Input: part model. Units: mm. Frame: model coordinates. Coordinates: 2 decimals unless noted, no trailing zeros. Loops run counter-clockwise (first coordinate to the right, second up) from the corner with the lowest first, then second, coordinate; pieces in that order, holes last. Notation, with made-up numbers: (68, -14.5) - (93, -14.5) arc R35 ccw to (93, 17.5) - close; hole circle Ø5 at (57.5, 44.5). An arc over 180 degrees is marked (long way). Use one line per item in the form item = value.
from build123d import *

# Parameters (mm, degrees)
BOSS_EXTRUDE1_DEPTH          = 1
CUT_EXTRUDE1_REACH           = 153.019
SKETCH2_R                    = 5.25
LPATTERN1_COUNT              = 6
LPATTERN1_PITCH              = 20
CIRPATTERN1_COPY_1_REACH     = 153.019
CIRPATTERN1_COPY_1_SKETCH_R  = 5.25
CIRPATTERN1_COPY_2_REACH     = 153.019
CIRPATTERN1_COPY_2_SKETCH_R  = 5.25
CIRPATTERN1_COPY_3_REACH     = 153.019
CIRPATTERN1_COPY_3_SKETCH_R  = 5.25
CIRPATTERN1_COPY_4_REACH     = 153.019
CIRPATTERN1_COPY_4_SKETCH_R  = 5.25
CIRPATTERN1_COPY_5_REACH     = 153.019
CIRPATTERN1_COPY_5_SKETCH_R  = 5.25
CIRPATTERN1_COPY_6_REACH     = 153.019
CIRPATTERN1_COPY_6_SKETCH_R  = 5.25
CIRPATTERN1_COPY_7_REACH     = 153.019
CIRPATTERN1_COPY_7_SKETCH_R  = 5.25
CIRPATTERN1_COPY_8_REACH     = 153.019
CIRPATTERN1_COPY_8_SKETCH_R  = 5.25
CIRPATTERN1_COPY_9_REACH     = 153.019
CIRPATTERN1_COPY_9_SKETCH_R  = 5.25
CIRPATTERN1_COPY_10_REACH    = 153.019
CIRPATTERN1_COPY_10_SKETCH_R = 5.25


with BuildPart() as part:
    # Sketch1 → Boss-Extrude1 (new, symmetric)
    with BuildSketch(Plane(origin=(0, 0, 0), x_dir=(1, 0, 0), z_dir=(0, 1, 0))):
        with BuildLine():
            ThreePointArc((-92.270407539, -35.95451472), (-97.990380878, -56.574773191), (-77.272726285, -61.931259218))
            ThreePointArc((-77.272726285, -61.931259218), (-7.65e-07, -40.496129118), (77.272724973, -61.931258429))
            ThreePointArc((77.272724973, -61.931258429), (97.990379986, -56.574774736), (92.270409321, -35.954515707))
            ThreePointArc((92.270409321, -35.954515707), (35.070677387, 20.248063146), (14.99768062, 97.88577308))
            ThreePointArc((14.99768062, 97.88577308), (9.1e-08, 113.149545762), (-14.997680623, 97.885773262))
            ThreePointArc((-14.997680623, 97.885773262), (-35.070676832, 20.248064107), (-92.270407539, -35.95451472))
        make_face()
    extrude(amount=BOSS_EXTRUDE1_DEPTH, both=True)

    # Sketch2 → Cut-Extrude1 (cut, up to next)
    with BuildSketch(Plane(origin=(0, 1, 0), x_dir=(1, 0, 0), z_dir=(0, 1, 0)), mode=Mode.PRIVATE) as cut_extrude1_sk1:
        with Locations(Location((0, 0, 0), (0, 0, 270))):
            Circle(SKETCH2_R)
    cut_extrude1_tool1 = extrude(cut_extrude1_sk1.sketch, amount=-CUT_EXTRUDE1_REACH, mode=Mode.PRIVATE) & part.part
    cut_extrude1 = cut_extrude1_tool1.solids().sort_by_distance((0, 1, 0))[0]
    add(cut_extrude1, mode=Mode.SUBTRACT)

    # LPattern1: Cut-Extrude1 ×6
    with Locations(*[(0, 0, -i * LPATTERN1_PITCH) for i in range(1, LPATTERN1_COUNT)]):
        add(cut_extrude1, mode=Mode.SUBTRACT)

    # CirPattern1 copy 1 sketch → CirPattern1 copy 1 (cut, up to next)
    with BuildSketch(Plane(origin=(-17.320508076, 1, 10), x_dir=(-0.4999999999999998, 0, -0.8660254037844387), z_dir=(0, 1, 0)), mode=Mode.PRIVATE) as cirpattern1_copy_1_sk1:
        with Locations(Location((0, 0, 0), (0, 0, 270))):
            Circle(CIRPATTERN1_COPY_1_SKETCH_R)
    cirpattern1_copy_1_tool1 = extrude(cirpattern1_copy_1_sk1.sketch, amount=-CIRPATTERN1_COPY_1_REACH, mode=Mode.PRIVATE) & part.part
    add(cirpattern1_copy_1_tool1.solids().sort_by_distance((-17.320508076, 1, 10))[0], mode=Mode.SUBTRACT)

    # CirPattern1 copy 2 sketch → CirPattern1 copy 2 (cut, up to next)
    with BuildSketch(Plane(origin=(17.320508076, 1, 10), x_dir=(-0.5000000000000004, 0, 0.8660254037844384), z_dir=(0, 1, 0)), mode=Mode.PRIVATE) as cirpattern1_copy_2_sk1:
        with Locations(Location((0, 0, 0), (0, 0, 270))):
            Circle(CIRPATTERN1_COPY_2_SKETCH_R)
    cirpattern1_copy_2_tool1 = extrude(cirpattern1_copy_2_sk1.sketch, amount=-CIRPATTERN1_COPY_2_REACH, mode=Mode.PRIVATE) & part.part
    add(cirpattern1_copy_2_tool1.solids().sort_by_distance((17.320508076, 1, 10))[0], mode=Mode.SUBTRACT)

    # CirPattern1 copy 3 sketch → CirPattern1 copy 3 (cut, up to next)
    with BuildSketch(Plane(origin=(-34.641016151, 1, 20), x_dir=(-0.4999999999999998, 0, -0.8660254037844387), z_dir=(0, 1, 0)), mode=Mode.PRIVATE) as cirpattern1_copy_3_sk1:
        with Locations(Location((0, 0, 0), (0, 0, 270))):
            Circle(CIRPATTERN1_COPY_3_SKETCH_R)
    cirpattern1_copy_3_tool1 = extrude(cirpattern1_copy_3_sk1.sketch, amount=-CIRPATTERN1_COPY_3_REACH, mode=Mode.PRIVATE) & part.part
    add(cirpattern1_copy_3_tool1.solids().sort_by_distance((-34.641016151, 1, 20))[0], mode=Mode.SUBTRACT)

    # CirPattern1 copy 4 sketch → CirPattern1 copy 4 (cut, up to next)
    with BuildSketch(Plane(origin=(34.641016151, 1, 20), x_dir=(-0.5000000000000004, 0, 0.8660254037844384), z_dir=(0, 1, 0)), mode=Mode.PRIVATE) as cirpattern1_copy_4_sk1:
        with Locations(Location((0, 0, 0), (0, 0, 270))):
            Circle(CIRPATTERN1_COPY_4_SKETCH_R)
    cirpattern1_copy_4_tool1 = extrude(cirpattern1_copy_4_sk1.sketch, amount=-CIRPATTERN1_COPY_4_REACH, mode=Mode.PRIVATE) & part.part
    add(cirpattern1_copy_4_tool1.solids().sort_by_distance((34.641016151, 1, 20))[0], mode=Mode.SUBTRACT)

    # CirPattern1 copy 5 sketch → CirPattern1 copy 5 (cut, up to next)
    with BuildSketch(Plane(origin=(-51.961524227, 1, 30), x_dir=(-0.4999999999999998, 0, -0.8660254037844387), z_dir=(0, 1, 0)), mode=Mode.PRIVATE) as cirpattern1_copy_5_sk1:
        with Locations(Location((0, 0, 0), (0, 0, 270))):
            Circle(CIRPATTERN1_COPY_5_SKETCH_R)
    cirpattern1_copy_5_tool1 = extrude(cirpattern1_copy_5_sk1.sketch, amount=-CIRPATTERN1_COPY_5_REACH, mode=Mode.PRIVATE) & part.part
    add(cirpattern1_copy_5_tool1.solids().sort_by_distance((-51.961524227, 1, 30))[0], mode=Mode.SUBTRACT)

    # CirPattern1 copy 6 sketch → CirPattern1 copy 6 (cut, up to next)
    with BuildSketch(Plane(origin=(51.961524227, 1, 30), x_dir=(-0.5000000000000004, 0, 0.8660254037844384), z_dir=(0, 1, 0)), mode=Mode.PRIVATE) as cirpattern1_copy_6_sk1:
        with Locations(Location((0, 0, 0), (0, 0, 270))):
            Circle(CIRPATTERN1_COPY_6_SKETCH_R)
    cirpattern1_copy_6_tool1 = extrude(cirpattern1_copy_6_sk1.sketch, amount=-CIRPATTERN1_COPY_6_REACH, mode=Mode.PRIVATE) & part.part
    add(cirpattern1_copy_6_tool1.solids().sort_by_distance((51.961524227, 1, 30))[0], mode=Mode.SUBTRACT)

    # CirPattern1 copy 7 sketch → CirPattern1 copy 7 (cut, up to next)
    with BuildSketch(Plane(origin=(-69.282032303, 1, 40), x_dir=(-0.4999999999999998, 0, -0.8660254037844387), z_dir=(0, 1, 0)), mode=Mode.PRIVATE) as cirpattern1_copy_7_sk1:
        with Locations(Location((0, 0, 0), (0, 0, 270))):
            Circle(CIRPATTERN1_COPY_7_SKETCH_R)
    cirpattern1_copy_7_tool1 = extrude(cirpattern1_copy_7_sk1.sketch, amount=-CIRPATTERN1_COPY_7_REACH, mode=Mode.PRIVATE) & part.part
    add(cirpattern1_copy_7_tool1.solids().sort_by_distance((-69.282032303, 1, 40))[0], mode=Mode.SUBTRACT)

    # CirPattern1 copy 8 sketch → CirPattern1 copy 8 (cut, up to next)
    with BuildSketch(Plane(origin=(69.282032303, 1, 40), x_dir=(-0.5000000000000004, 0, 0.8660254037844384), z_dir=(0, 1, 0)), mode=Mode.PRIVATE) as cirpattern1_copy_8_sk1:
        with Locations(Location((0, 0, 0), (0, 0, 270))):
            Circle(CIRPATTERN1_COPY_8_SKETCH_R)
    cirpattern1_copy_8_tool1 = extrude(cirpattern1_copy_8_sk1.sketch, amount=-CIRPATTERN1_COPY_8_REACH, mode=Mode.PRIVATE) & part.part
    add(cirpattern1_copy_8_tool1.solids().sort_by_distance((69.282032303, 1, 40))[0], mode=Mode.SUBTRACT)

    # CirPattern1 copy 9 sketch → CirPattern1 copy 9 (cut, up to next)
    with BuildSketch(Plane(origin=(-86.602540378, 1, 50), x_dir=(-0.4999999999999998, 0, -0.8660254037844387), z_dir=(0, 1, 0)), mode=Mode.PRIVATE) as cirpattern1_copy_9_sk1:
        with Locations(Location((0, 0, 0), (0, 0, 270))):
            Circle(CIRPATTERN1_COPY_9_SKETCH_R)
    cirpattern1_copy_9_tool1 = extrude(cirpattern1_copy_9_sk1.sketch, amount=-CIRPATTERN1_COPY_9_REACH, mode=Mode.PRIVATE) & part.part
    add(cirpattern1_copy_9_tool1.solids().sort_by_distance((-86.602540378, 1, 50))[0], mode=Mode.SUBTRACT)

    # CirPattern1 copy 10 sketch → CirPattern1 copy 10 (cut, up to next)
    with BuildSketch(Plane(origin=(86.602540378, 1, 50), x_dir=(-0.5000000000000004, 0, 0.8660254037844384), z_dir=(0, 1, 0)), mode=Mode.PRIVATE) as cirpattern1_copy_10_sk1:
        with Locations(Location((0, 0, 0), (0, 0, 270))):
            Circle(CIRPATTERN1_COPY_10_SKETCH_R)
    cirpattern1_copy_10_tool1 = extrude(cirpattern1_copy_10_sk1.sketch, amount=-CIRPATTERN1_COPY_10_REACH, mode=Mode.PRIVATE) & part.part
    add(cirpattern1_copy_10_tool1.solids().sort_by_distance((86.602540378, 1, 50))[0], mode=Mode.SUBTRACT)


solid = part.part
Q1. First-contact query: P1, Ø6.5, axis at x = 0, z = -80, coming from the +Y side. Flat tip, straight axial feed; report the tip coordinate or a pass-through.
Check values:
P1 = through
Q2. Pull-direction query (X, two-part tool) for faces 1 (the cylindrical face through (52.192, 0.014, 24.755)), 2 (the flat face through (-8, -1, -5)), 3 (the cylindrical face through (0.334, 0.014, -113.146)); classes: pulls with the +X half, pulls with the -X half, needs draft (parallel to the pull), parting line crosses it, or undercut.
Check values:
face_1 = undercut
face_2 = needs draft
face_3 = parting line crosses it
Q3. Cut plane A-A, the plane x = 0. Return loops of the section in (y, z).
Check values:
outline = (-1, -113.15) - (1, -113.15) - (1, -105.25) - (-1, -105.25) - close; (-1, -94.75) - (1, -94.75) - (1, -85.25) - (-1, -85.25) - close; (-1, -74.75) - (1, -74.75) - (1, -65.25) - (-1, -65.25) - close; (-1, -54.75) - (1, -54.75) - (1, -45.25) - (-1, -45.25) - close; (-1, -34.75) - (1, -34.75) - (1, -25.25) - (-1, -25.25) - close; (-1, -14.75) - (1, -14.75) - (1, -5.25) - (-1, -5.25) - close; (-1, 5.25) - (1, 5.25) - (1, 40.5) - (-1, 40.5) - close
Q4. Ray query, line 1 along X through (y, z) = (-0.1, 30); line 2 along Z through (x, y) = (-47.5, -0.6); line 3 along Z through (x, y) = (73.5, -0.2). Return the intervals inside material, ascending. Write a range as [from, to].
Check values:
line_1 = [-82.43, -57.21], [-46.71, 46.71], [57.21, 82.43]
line_2 = [-1.98, 27.23], [32.77, 48.22]
line_3 = [23.63, 36.87], [43.13, 59.74]
Q5. Cut plane D-D, the plane z = 21.5. Return loops of the section in (x, y), then the cut area to 3 significant figures.
Check values:
outline = (-70.79, -1) - (-39.67, -1) - (-39.67, 1) - (-70.79, 1) - close; (-29.61, -1) - (29.61, -1) - (29.61, 1) - (-29.61, 1) - close; (39.67, -1) - (70.79, -1) - (70.79, 1) - (39.67, 1) - close
area = 243 mm²
Q6. Cut plane B-B, the plane z = -61. Return loops of the section in (x, y).
Check values:
outline = (-18.94, -1) - (-5.15, -1) - (-5.15, 1) - (-18.94, 1) - close; (5.15, -1) - (18.94, -1) - (18.94, 1) - (5.15, 1) - close
Q7. Cut plane C-C, the plane y = 0. Give the number of separate pieces and of enclosed holes in the cut face, then the cut area to 3 significant figures.
Check values:
separate_pieces = 1
enclosed_holes = 16
area = 11,700 mm²
